Geometry check sheet. Reference: the model listing, model coordinates, mm. A direction names the side the tool comes from. Give positions to 0.01 mm unless a question says otherwise; leave off trailing zeros. Order: outer loops, then holes, each group sorted by start corner. A loop starts at its lowest first (then second) coordinate and runs counter-clockwise, first axis right, second up. Notation, with made-up numbers: M 30.5,70.25 L 69.5,70.25 A25 cw 69.5,103.25 Z; hole C -14,53 d10. An arc over 180 degrees is marked long. Answer as CSV lines item,"result".
from build123d import *

# Parameters (mm, degrees)
SKETCH1_R                      = 3.925
SKETCH1_R_2                    = 2.924999992
BOSS_EXTRUDE1_DEPTH            = 4
SKETCH1_R_3                    = 0.875
BOSS_EXTRUDE1_2_DEPTH          = 4
SKETCH2_W                      = 20
SKETCH2_H                      = 15
BOSS_EXTRUDE2_DEPTH            = 3
BOSS_EXTRUDE3_START            = 10
SKETCH3_W                      = 15
SKETCH3_H                      = 50
BOSS_EXTRUDE3_DEPTH            = 3
F_3_2_3_2_DIAMETER_HOLE1_D     = 3.2
F_3_2_3_2_DIAMETER_HOLE1_DEPTH = 4
F_3_2_3_2_DIAMETER_HOLE1_TIP   = 0.96137699


with BuildPart() as part:
    # Sketch1 → Boss-Extrude1 (new body)
    with BuildSketch(Plane(origin=(0, 0, 0), x_dir=(1, 0, 0), z_dir=(0, 1, 0))):
        with Locations(Location((0, 0, 0), (0, 0, 270))):
            Circle(SKETCH1_R)
        with Locations(Location((0, 0, 0), (0, 0, 270))):
            Circle(SKETCH1_R_2, mode=Mode.SUBTRACT)
    extrude(amount=BOSS_EXTRUDE1_DEPTH)



with BuildPart() as body_2:
    # Sketch1 → Boss-Extrude1 2 (new body)
    with BuildSketch(Plane(origin=(0, 0, 0), x_dir=(1, 0, 0), z_dir=(0, 1, 0))):
        with Locations(Location((0, 0, 0), (0, 0, 270))):
            Circle(SKETCH1_R_3)
    extrude(amount=BOSS_EXTRUDE1_2_DEPTH)


with BuildPart() as part_1:
    add(part.part)

    add(body_2.part)  # Boss-Extrude2 merges body 2
    # Sketch2 → Boss-Extrude2 (add)
    with BuildSketch(Plane(origin=(0, 4, 0), x_dir=(1, 0, 0), z_dir=(0, 1, 0))):
        Rectangle(SKETCH2_W, SKETCH2_H)
    extrude(amount=BOSS_EXTRUDE2_DEPTH)

    # Sketch3 → Boss-Extrude3 (add)
    with BuildSketch(Plane(origin=(0, 0, 0), x_dir=(0, 0, -1), z_dir=(1, 0, 0)).offset(BOSS_EXTRUDE3_START)):
        with Locations((0, 29)):
            Rectangle(SKETCH3_W, SKETCH3_H)
    extrude(amount=-BOSS_EXTRUDE3_DEPTH)

    # Ø3.2 (3.2) Diameter Hole1
    with Locations(Plane(origin=(10, 0, 0), x_dir=(0, 0, -1), z_dir=(1, 0, 0))):
        with Locations((0, 12), (0, 49)):
            Hole(F_3_2_3_2_DIAMETER_HOLE1_D / 2, depth=F_3_2_3_2_DIAMETER_HOLE1_DEPTH)
            with Locations((0, 0, -(F_3_2_3_2_DIAMETER_HOLE1_DEPTH + F_3_2_3_2_DIAMETER_HOLE1_TIP / 2))):  # 118° drill point
                Cone(0, F_3_2_3_2_DIAMETER_HOLE1_D / 2, F_3_2_3_2_DIAMETER_HOLE1_TIP, mode=Mode.SUBTRACT)


solid = part_1.part
(1) Section check B-B on y = 12. Enter the section's corners in (x, z).
The answers:
outline,"M 7,-7.5 L 10,-7.5 L 10,-1.6 L 7,-1.6 Z; M 7,1.6 L 10,1.6 L 10,7.5 L 7,7.5 Z"
(2) Tool access check on faces 1 (the face through (8.479, 13.586, -0.208)), 2 (the face through (1, 4, -1)), 3 (the face through (7, 31, 0)). Record the directions out of +Z, -Z, +X, -X, +Y, -Y that give a thin tool (end or side, any length) a straight path to the whole face; none if there is none.
The answers:
face 1,"+X, -X"
face 2,"-Y"
face 3,"+Z, -Z, -X, +Y"
(3) Section check A-A on z = 0. Enter the section's corners in (x, y) (3 decimals), then the cut area to 3 significant figures.
The answers:
outline,"M -10,4 L -3.925,4 L -3.925,0 L -2.925,0 L -2.925,4 L -0.875,4 L -0.875,0 L 0.875,0 L 0.875,4 L 2.925,4 L 2.925,0 L 3.925,0 L 3.925,4 L 10,4 L 10,10.4 L 7,10.4 L 7,7 L -10,7 Z; M 7,13.6 L 10,13.6 L 10,47.4 L 7,47.4 Z; M 7,50.6 L 10,50.6 L 10,54 L 7,54 Z"
area,"197 mm2"
(4) Section check C-C on x = 0. Enter the section's corners in (y, z) (3 decimals), then the cut area to 3 significant figures.
The answers:
outline,"M 0,-3.925 L 4,-3.925 L 4,-7.5 L 7,-7.5 L 7,7.5 L 4,7.5 L 4,3.925 L 0,3.925 L 0,2.925 L 4,2.925 L 4,0.875 L 0,0.875 L 0,-0.875 L 4,-0.875 L 4,-2.925 L 0,-2.925 Z"
area,"60.0 mm2"
(5) Gauge pin test, flat ends, axial feed: P1, Ø1, axis at y = 22.5, z = -1.5, coming from the -X side; P2, Ø7.5, axis at x = 2, z = 1.5, coming from the +Y side. Record the tip position at first contact, or that the pin passes through.
The answers:
P1,"stops at x = 7"
P2,"stops at y = 7"
(6) Draft check along X on faces 4 (the face through (-2, 7, 0)), 5 (the face through (0.88, 1.97, 2.79)), 6 (the face through (-10, 5, 0)), 7 (the face through (10, 29, 0)). Enter one of: +X half, -X half, draft (parallel to the pull), parting line (faces both ways), or undercut.
The answers:
face 4,"draft"
face 5,"undercut"
face 6,"-X half"
face 7,"+X half"
(7) Section check D-D on z = 6.5. Enter the section's corners in (x, y), then the cut area to 3 significant figures.
The answers:
outline,"M -10,4 L 10,4 L 10,54 L 7,54 L 7,7 L -10,7 Z"
area,"201 mm2"
(8) Material ranges on line 1 (Y direction, x = 8.4, z = 0); line 2 (X direction, y = 0.9, z = 0) (3 decimals); line 3 (X direction, y = 39, z = -3.5), recorded low to high.
The answers:
line 1,"y = 4 to 10.4, 13.6 to 47.4, 50.6 to 54"
line 2,"x = -3.925 to -2.925, -0.875 to 0.875, 2.925 to 3.925"
line 3,"x = 7 to 10"
